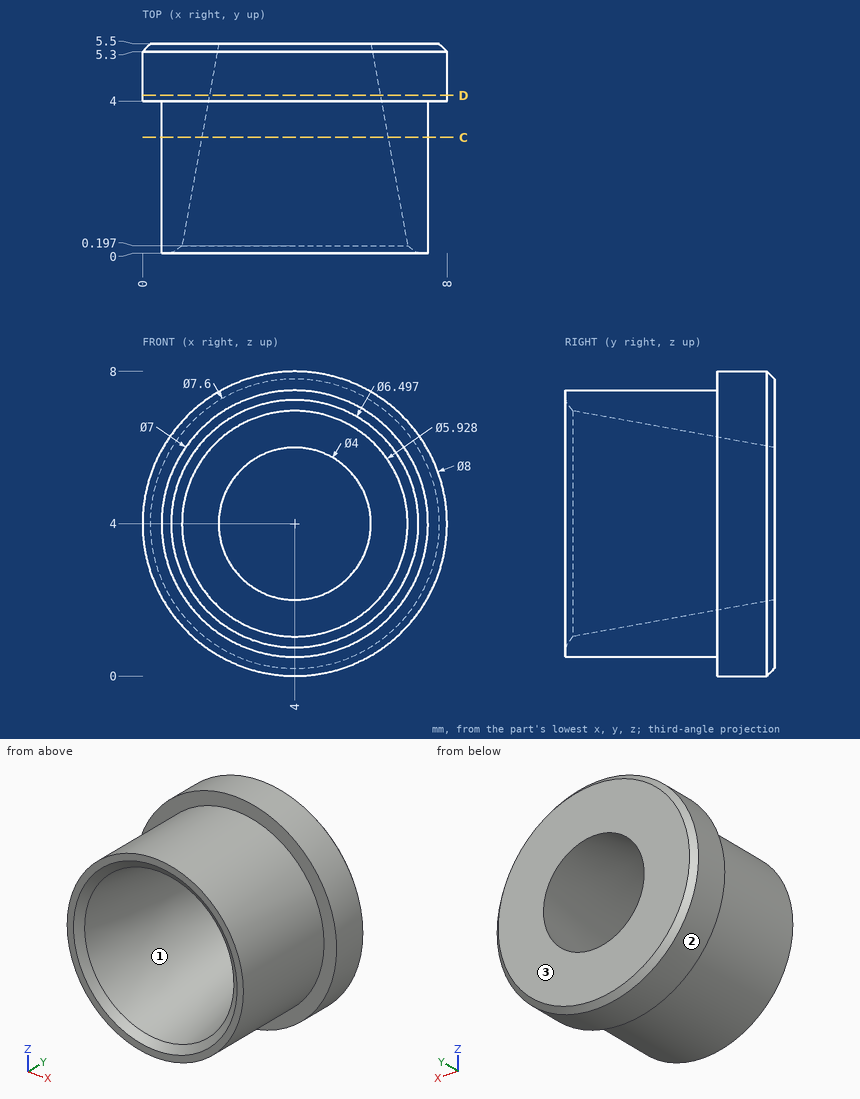
Input: dimensioned drawing with shaded views. Units: mm. Origin: part minimum x, y, z. Round coordinates to 2 decimals unless told otherwise and drop trailing zeros. Order: outer loops, then holes, each group sorted by start corner. A loop starts at its lowest first (then second) coordinate and runs counter-clockwise, first axis right, second up.
Q1. Mould query, pull axis Z, two halves, no side actions, for the marked faces 1, 2 and 3. Classes: released by +Z, released by -Z, zero draft, split by the parting line, or undercut.
Result sheet:
face 1: undercut
face 2: split by the parting line
face 3: zero draft
Q2. Material intervals for probe 1 along X at (y, z) = (1.6, 6) (1 decimal); probe 2 along X at (y, z) = (2.6, 6) (1 decimal); probe 3 along Z at (x, y) = (2, 3.25) (1 decimal), sorted ascending.
Result sheet:
probe 1: x = 1.1 to 2.2, 5.8 to 6.9
probe 2: x = 1.1 to 2.5, 5.5 to 6.9
probe 3: z = 1.1 to 2.7, 5.3 to 6.9
Q3. Section C-C, the plane y = 3.05. Output: boundary loops of the cut face in (x, z) (1 decimal).
Result sheet:
outline: circle Ø7 at (4, 4); hole circle Ø4.9 at (4, 4)
Q4. Pin query (flat end, axial travel): pin 1 (1.5 mm diameter, centred on x = 3, y = 4.5, fed in from +Z); pin 2 (1.5 mm diameter, centred on x = 6.5, y = 1.5, fed in from +Z). Return the tip coordinate at first contact, or that it passes through.
Result sheet:
pin 1: stops at z = 7.99
pin 2: stops at z = 7.03
Q5. Section D-D, the plane y = 4.15. Output: boundary loops of the cut face in (x, z) (1 decimal).
Result sheet:
outline: circle Ø8 at (4, 4); hole circle Ø4.5 at (4, 4)
